```python
from build123d import *

# Parameters (mm, degrees)
ESQUISSE1_W        = 140
ESQUISSE1_H        = 100
ESQUISSE1_R        = 1.55
BOSS_EXTRU_1_DEPTH = 5


with BuildPart() as part:
    # Esquisse1 → Boss.-Extru.1 (new body)
    with BuildSketch(Plane.XY):
        Rectangle(ESQUISSE1_W, ESQUISSE1_H)
        with Locations((-60, -40)):
            Circle(ESQUISSE1_R, mode=Mode.SUBTRACT)
        with Locations(Location((60, -40, 0), (0, 0, 180))):
            Circle(ESQUISSE1_R, mode=Mode.SUBTRACT)
        with Locations((60, 40)):
            Circle(ESQUISSE1_R, mode=Mode.SUBTRACT)
        with Locations(Location((-60, 40, 0), (0, 0, 180))):
            Circle(ESQUISSE1_R, mode=Mode.SUBTRACT)
    extrude(amount=-BOSS_EXTRU_1_DEPTH)


solid = part.part
```
Here's how the part is built. I have some questions about the finished solid (model axes, mm). Coordinates: 2 decimals unless noted, no trailing zeros. Order: outer loops, then holes, each group sorted by start corner. A loop starts at its lowest first (then second) coordinate and runs counter-clockwise, first axis right, second up. Notation, with made-up numbers: (-10.75, 32.5) -> (27.25, 32.5) arc R36 cw to (27.25, 71.5) -> close; hole circle Ø2 at (66.25, 67). An arc over 180 degrees is marked (long way). Return JSON: item names as keys, results as strings.
1) Thinking about a two-plate mould opening in X: for faces 1 (the flat face through (-1, 1, -5)), 2 (the flat face through (-70, -1, -2)), 3 (the flat face through (70, -1, -2)), 4 (the cylindrical face through (-58.568, -40.594, -2.465)), which applies, +X half, -X half, draft (parallel to the pull), parting line (faces both ways), or undercut?
Conclusion:
{"face 1": "draft", "face 2": "-X half", "face 3": "+X half", "face 4": "undercut"}
2) If we section it at B-B on x = 60: List the corners of the cut face in (y, z) for me, plus the area to 3 significant figures.
Conclusion:
{"outline": "(-50, -5) -> (-41.55, -5) -> (-41.55, 0) -> (-50, 0) -> close; (-38.45, -5) -> (38.45, -5) -> (38.45, 0) -> (-38.45, 0) -> close; (41.55, -5) -> (50, -5) -> (50, 0) -> (41.55, 0) -> close", "area": "469 mm²"}
3) If we section it at A-A on y = -40: List the corners of the cut face in (x, z) for me, plus the area to 3 significant figures.
Conclusion:
{"outline": "(-70, -5) -> (-61.55, -5) -> (-61.55, 0) -> (-70, 0) -> close; (-58.45, -5) -> (58.45, -5) -> (58.45, 0) -> (-58.45, 0) -> close; (61.55, -5) -> (70, -5) -> (70, 0) -> (61.55, 0) -> close", "area": "669 mm²"}
4) If I drill on probe 1 along Y at (x, z) = (-60, -3.9); probe 2 along Y at (x, z) = (61, -2.3); probe 3 along X at (y, z) = (-39.5, -2.9), over which ranges is the centre line in solid material (lowest first)?
Conclusion:
{"probe 1": "y = -50 to -41.55, -38.45 to 38.45, 41.55 to 50", "probe 2": "y = -50 to -41.18, -38.82 to 38.82, 41.18 to 50", "probe 3": "x = -70 to -61.47, -58.53 to 58.53, 61.47 to 70"}
